from build123d import *

# Parameters (mm, degrees)
F0_W     = 2440
F0_H     = 1220
F1_DEPTH = 54
F0_W_2   = 202
F0_H_2   = 814
F2_DEPTH = 54
F0_W_3   = 916
F3_DEPTH = 18


with BuildPart() as f1:
    # F0 (on Top) → F1 (new body)
    with BuildSketch(Plane.XY):
        with Locations((-1220, 610)):
            Rectangle(F0_W, F0_H)
        Polygon((-2237, 203), (-2237, 1017), (-1321, 1017), (-1119, 1017), (-203, 1017), (-203, 203), (-1119, 203), (-1321, 203), align=None, mode=Mode.SUBTRACT)
    extrude(amount=F1_DEPTH)

    # F0 (on Top) → F2 (join)
    with BuildSketch(Plane.XY):
        with Locations((-1220, 610)):
            Rectangle(F0_W_2, F0_H_2)
    extrude(amount=F2_DEPTH)

    # F0 (on Top) → F3 (join)
    with BuildSketch(Plane.XY):
        with Locations((-1779, 610)):
            Rectangle(F0_W_3, F0_H_2)
        with Locations((-661, 610)):
            Rectangle(F0_W_3, F0_H_2)
    extrude(amount=F3_DEPTH)


solid = f1.part
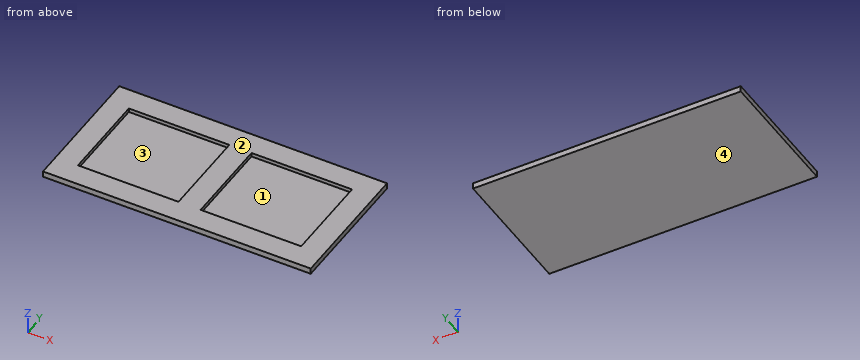
Here's how the part is built. I have some questions about the finished solid (model axes, mm). Face numbers are marked on the shaded views. A direction names the side the tool comes from. Give positions to 0.01 mm unless a question says otherwise; leave off trailing zeros. Order: outer loops, then holes, each group sorted by start corner. A loop starts at its lowest first (then second) coordinate and runs counter-clockwise, first axis right, second up. Notation, with made-up numbers: (-30.75, 53.5) -> (19.25, 53.5) arc R20 cw to (19.25, 71.5) -> close; hole circle Ø11 at (79, 60.25). An arc over 180 degrees is marked (long way). One line per item, written item: value. Start each with the question number.
1. Imagine slicing it at C-C, the plane y = 830.5. List the corners of the cut face in (x, z) for me, plus the area to 3 significant figures.
2. Imagine slicing it at A-A, the plane z = 44.5. List the corners of the cut face in (x, y) for me, plus the area to 3 significant figures.
3. For the marked faces 3 and 4, which set-ups out of +Z, -Z, +X, -X, +Y, -Y let a thin tool reach every point of the face, with its end or its side?
4. I need wall thicknesses on probe 1 along X at (y, z) = (460, 26); probe 2 along Y at (x, z) = (-2090, 42); probe 3 along Z at (x, y) = (-1809.5, 636). Which ranges of each line are inside material? Lowest first, please. Write a range as from..to.
5. Will this pin go through, and if not, where does the flat tip stop? pin 1 Ø4 at (x, y) = (-1423.5, 238) entering from +Z.
6. Imagine slicing it at B-B, the plane x = -2104. List the corners of the cut face in (y, z) for me, plus the area to 3 significant figures.
7. We'd pull the mould along X, two halves only. Please class the marked faces 1 and 2: released by +X, released by -X, zero draft, split by the parting line, or undercut.
Values follow:
1. outline: (-2440, 0) -> (0, 0) -> (0, 54) -> (-203, 54) -> (-203, 18) -> (-1119, 18) -> (-1119, 54) -> (-1321, 54) -> (-1321, 18) -> (-2237, 18) -> (-2237, 54) -> (-2440, 54) -> close
1. area: 65,800 mm2
2. outline: (-2440, 0) -> (0, 0) -> (0, 1220) -> (-2440, 1220) -> close; hole (-2237, 203) -> (-1321, 203) -> (-1321, 1017) -> (-2237, 1017) -> close; hole (-1119, 203) -> (-203, 203) -> (-203, 1017) -> (-1119, 1017) -> close
2. area: 1,490,000 mm2
3. face 3: +Z
3. face 4: -Z, +X, -X, +Y, -Y
4. probe 1: x = -2440..-2237, -1321..-1119, -203..0
4. probe 2: y = 0..203, 1017..1220
4. probe 3: z = 0..18
5. pin 1: stops at z = 18
6. outline: (0, 0) -> (1220, 0) -> (1220, 54) -> (1017, 54) -> (1017, 18) -> (203, 18) -> (203, 54) -> (0, 54) -> close
6. area: 36,600 mm2
7. face 1: undercut
7. face 2: zero draft
